```python
from build123d import *

# Parameters (mm, degrees)
F1_DEPTH = 38.1
F2_R     = 9.525
F3_DEPTH = 76.2
F5_DEPTH = 50.8


# Not quite as in the source:
# - a feature names something its author has since deleted; it is built from what else it names


with BuildPart() as f1:
    # F0 (on Front) → F1 (new body)
    with BuildSketch(Plane.XZ):
        with BuildLine():
            Line((1.4605, 7.5692852344), (1.4605, 9.3218852344))
            Line((1.4605, 9.3218852344), (-1.4605, 9.3218852344))
            Line((-1.4605, 9.3218852344), (-1.4605, 7.5692852344))
            ThreePointArc((-1.4605, 7.5692852344), (-2.2699762391, 6.9862685009), (-3.2675449109, 6.9821407509))
            Line((-3.2675449109, 6.9821407509), (-4.2976973441, 8.4000239352))
            Line((-4.2976973441, 8.4000239352), (-6.6608359846, 6.6831032133))
            Line((-6.6608359846, 6.6831032133), (-5.6306835515, 5.2652200289))
            ThreePointArc((-5.6306835515, 5.2652200289), (-5.9428749476, 4.3177513881), (-6.7474987256, 3.7280558148))
            Line((-6.7474987256, 3.7280558148), (-8.4143203761, 4.2696389991))
            Line((-8.4143203761, 4.2696389991), (-9.3169590166, 1.491602915))
            Line((-9.3169590166, 1.491602915), (-7.6501373662, 0.9500197307))
            ThreePointArc((-7.6501373662, 0.9500197307), (-7.3457974171, 0), (-7.6501373662, -0.9500197307))
            Line((-7.6501373662, -0.9500197307), (-9.3169590166, -1.491602915))
            Line((-9.3169590166, -1.491602915), (-8.4143203761, -4.2696389991))
            Line((-8.4143203761, -4.2696389991), (-6.7474987256, -3.7280558148))
            ThreePointArc((-6.7474987256, -3.7280558148), (-5.9428749476, -4.3177513881), (-5.6306835515, -5.2652200289))
            Line((-5.6306835515, -5.2652200289), (-6.6608359846, -6.6831032133))
            Line((-6.6608359846, -6.6831032133), (-4.2976973441, -8.4000239352))
            Line((-4.2976973441, -8.4000239352), (-3.2675449109, -6.9821407509))
            ThreePointArc((-3.2675449109, -6.9821407509), (-2.2699762391, -6.9862685009), (-1.4605, -7.5692852344))
            Line((-1.4605, -7.5692852344), (-1.4605, -9.3218852344))
            Line((-1.4605, -9.3218852344), (1.4605, -9.3218852344))
            Line((1.4605, -9.3218852344), (1.4605, -7.5692852344))
            ThreePointArc((1.4605, -7.5692852344), (2.2699762391, -6.9862685009), (3.2675449109, -6.9821407509))
            Line((3.2675449109, -6.9821407509), (4.2976973441, -8.4000239352))
            Line((4.2976973441, -8.4000239352), (6.6608359846, -6.6831032133))
            Line((6.6608359846, -6.6831032133), (5.6306835515, -5.2652200289))
            ThreePointArc((5.6306835515, -5.2652200289), (5.9428749476, -4.3177513881), (6.7474987256, -3.7280558148))
            Line((6.7474987256, -3.7280558148), (8.4143203761, -4.2696389991))
            Line((8.4143203761, -4.2696389991), (9.3169590166, -1.491602915))
            Line((9.3169590166, -1.491602915), (7.6501373662, -0.9500197307))
            ThreePointArc((7.6501373662, -0.9500197307), (7.3457974171, 0), (7.6501373662, 0.9500197307))
            Line((7.6501373662, 0.9500197307), (9.3169590166, 1.491602915))
            Line((9.3169590166, 1.491602915), (8.4143203761, 4.2696389991))
            Line((8.4143203761, 4.2696389991), (6.7474987256, 3.7280558148))
            ThreePointArc((6.7474987256, 3.7280558148), (5.9428749476, 4.3177513881), (5.6306835515, 5.2652200289))
            Line((5.6306835515, 5.2652200289), (6.6608359846, 6.6831032133))
            Line((6.6608359846, 6.6831032133), (4.2976973441, 8.4000239352))
            Line((4.2976973441, 8.4000239352), (3.2675449109, 6.9821407509))
            ThreePointArc((3.2675449109, 6.9821407509), (2.2699762391, 6.9862685009), (1.4605, 7.5692852344))
        make_face()
    extrude(amount=F1_DEPTH)

    # F2 (on Front) → F3 (join)
    with BuildSketch(Plane.XZ):
        Circle(F2_R)
    extrude(amount=-F3_DEPTH)

    # F4 (on face) → F5 (cut)
    with BuildSketch(Plane(origin=(0, 76.2, 0), x_dir=(-1, 0, 0), z_dir=(0, 1, 0))):
        with BuildLine():
            ThreePointArc((2.38125, 9.2225415932), (1.2001908859, 9.4490828569), (0, 9.525))
            ThreePointArc((0, 9.525), (-1.2001908859, 9.4490828569), (-2.38125, 9.2225415932))
            Line((-2.38125, 9.2225415932), (-2.38125, 6.8326))
            Line((-2.38125, 6.8326), (2.38125, 6.8326))
            Line((2.38125, 6.8326), (2.38125, 9.2225415932))
        make_face()
    extrude(amount=-F5_DEPTH, mode=Mode.SUBTRACT)


solid = f1.part
```
For this review, take the finished solid that the model builds, in its own axes (mm). A direction names the side the tool comes from. Coordinates: 2 decimals unless noted, no trailing zeros. Loops run counter-clockwise (first coordinate to the right, second up) from the corner with the lowest first, then second, coordinate; pieces in that order, holes last. Notation, with made-up numbers: (83.25, 11.25) -> (124.25, 11.25) arc R29 cw to (124.25, 41.25) -> close; hole circle Ø1 at (-35.5, 58.5). An arc over 180 degrees is marked (long way). Return JSON: item names as keys, results as strings. Group by question number.
(1) Consider section C-C, the plane y = 5.5. Give the boundary of the cut face in (x, z) (3 decimals).
(2) To check wall thickness, follow L1, parallel to X at y = -15, z = 8; L2, parallel to Y at x = 7.5, z = 5.75; L3, parallel to X at y = 48.5, z = -4.5. State the ranges of each line that lie inside material, in increasing order.
(3) Tool access review of faces 1 (the flat face through (-2.381, 51, 8)), 2 (the cylindrical face through (7.346, -18.783, -0.014)), 3 (the flat face through (8.86, -18.78, -2.9)), 4 (the flat face through (0, -19, 9.322)): name each direction out of +Z, -Z, +X, -X, +Y, -Y from which nothing blocks a thin tool from reaching the whole face with its end or side.
(4) Consider section A-A, the plane z = 0. Give the boundary of the cut face in (x, y) (3 decimals), plus the area to 3 significant figures.
(5) Consider section B-B, the plane x = 0. Give the boundary of the cut face in (y, z) (3 decimals).
(6) Mouldability with a two-part tool opening along X and no side actions: class faces 5 (the flat face through (0, -38.1, 0)), 6 (the cylindrical face through (2.26, -18.78, -6.99)), 7 (the flat face through (-8.872, -18.783, -2.861)) as pulls with the +X half, pulls with the -X half, needs draft (parallel to the pull), parting line crosses it, or undercut.
(7) For pin 1 Ø1.2 at (y, z) = (51.5, 8.5) entering from -X; pin 2 Ø4 at (y, z) = (2, 2.5) entering from -X; pin 3 Ø2.5 at (x, y) = (-1, 52) entering from +Z, all flat-tipped, find the tip position at first contact; note any pin that passes through.
(8) Consider section D-D, the plane y = 34. Give the boundary of the cut face in (x, z) (3 decimals), plus the area to 3 significant figures.
Results below:
{
 "1": {"outline": "circle Ø19.05 at (0, 0)"},
 "2": {"L1": "x = -4.85 to -4.01, -1.46 to 1.46, 4.01 to 4.85", "L2": "y = 0 to 76.2", "L3": "x = -8.39 to 8.39"},
 "3": {"face 1": "+Z, +Y", "face 2": "+X, -Y", "face 3": "-Z, +X, -Y", "face 4": "+Z, +X, -X, -Y"},
 "4": {"outline": "(-9.525, 0) -> (-7.346, 0) -> (-7.346, -38.1) -> (7.346, -38.1) -> (7.346, 0) -> (9.525, 0) -> (9.525, 76.2) -> (-9.525, 76.2) -> close", "area": "2,010 mm2"},
 "5": {"outline": "(-38.1, -9.322) -> (0, -9.322) -> (0, -9.525) -> (76.2, -9.525) -> (76.2, 6.833) -> (25.4, 6.833) -> (25.4, 9.525) -> (0, 9.525) -> (0, 9.322) -> (-38.1, 9.322) -> close"},
 "6": {"face 5": "needs draft", "face 6": "undercut", "face 7": "pulls with the -X half"},
 "7": {"pin 1": "stops at x = -5.32", "pin 2": "stops at x = -9.51", "pin 3": "stops at z = 6.83"},
 "8": {"outline": "(-2.381, 6.833) -> (-2.381, 9.223) arc R9.525 ccw (long way) to (2.381, 9.223) -> (2.381, 6.833) -> close", "area": "273 mm2"}
}
